Autodesk Inventor part; units mm, degrees
ref_plane "YZ Plane" through (0, 0, 0) normal (1, 0, 0) x (0, 1, 0)
ref_plane "XZ Plane" through (0, 0, 0) normal (0, 1, 0) x (-1, 0, 0)
ref_plane "XY Plane" through (0, 0, 0) normal (0, 0, 1) x (1, 0, 0)
ref_plane "Work Plane1" through (0, 0, 0) normal (0, 0, 1) x (1, 0, 0)
sketch "Sketch1" plane through (0, 0, 0) normal (0, 0, 1) x (1, 0, 0)
  line L0 (-150, -200) -> (150, -200)
  line L1 (150, -200) -> (150, 200)
  line L2 (150, 200) -> (-150, 200)
  line L3 (-150, 200) -> (-150, -200)
  line L4 (0, -280) -> (0, 280) construction
  line L5 (-210, 0) -> (210, 0) construction
  point P0 (0, 0)
  dimension "d0" = 400
  dimension "d1" = 300
extrude "Extrusion1" add sketch "Sketch1" against normal blind 12
sketch "Sketch2" plane through (0, 0, -12) normal (0, 0, 1) x (1, 0, 0)
  line L0 (0, 0) -> (-281.1142, 0) construction
  line L1 (0, 0) -> (0, -490.5016) construction
  line L2 (-150, -200) -> (150, -200) construction
  line L3 (-106.6853, -185) -> (102.3994, -185) construction
  line L4 (-96.6591, -157) -> (112.4256, -157) construction
  circle A0 centre (-82.5, -144) radius 2.15 construction
  circle A1 centre (-107.5, -144) radius 2.15 construction
  circle A2 centre (-107.5, 144) radius 2.15 construction
  circle A3 centre (-82.5, 144) radius 2.15 construction
  circle A4 centre (82.5, 144) radius 2.15 construction
  circle A5 centre (107.5, 144) radius 2.15 construction
  circle A6 centre (82.5, -144) radius 2.15 construction
  circle A7 centre (107.5, -144) radius 2.15 construction
  point P0 (-22.5, -157)
  point P1 (-34, -185)
  point P2 (22.5, -157)
  point P3 (34, -185)
  point P4 (-22.5, 157)
  point P5 (-34, 185)
  point P6 (34, 185)
  point P7 (22.5, 157)
  dimension "d8" = 15
  dimension "d9" = 28
  dimension "d10" = 22.5
  dimension "d11" = 34
hole "Hole2" at (-22.5, -157, -12) at (-34, -185, -12) at (34, -185, -12) at (22.5, -157, -12) at (-22.5, 157, -12) at (22.5, 157, -12) at (34, 185, -12) at (-34, 185, -12) at (107.5, -144, -12) at (82.5, -144, -12) at (-82.5, -144, -12) at (-107.5, -144, -12) at (-107.5, 144, -12) at (-82.5, 144, -12) at (82.5, 144, -12) at (107.5, 144, -12) direction (0, 0, 1) diameter 4.1 end through all counterbore diameter 7.2 counterbore depth 4.1
sketch "Sketch3" plane through (0, 0, -12) normal (0, 0, -1) x (-1, 0, 0)
  line L0 (-150, -200) -> (150, -200) construction
  line L1 (150, -200) -> (150, 200) construction
  line L2 (-150, 200) -> (-150, -200) construction
  line L3 (150, 200) -> (-150, 200) construction
  line L4 (135, -185) -> (-135, -185) construction
  line L5 (-135, -185) -> (-135, 185) construction
  line L6 (-135, 185) -> (135, 185) construction
  line L7 (135, 185) -> (135, -185) construction
  point P0 (0, 0)
  dimension "d29" = 15
hole "Hole3" at (-135, -185, -12) at (-135, 185, -12) at (135, 185, -12) at (135, -185, -12) direction (0, 0, 1) diameter 8.2 end through all
sketch "Sketch6" plane through (0, 0, -12) normal (0, 0, 1) x (1, 0, 0)
  line L0 (-27.5, -40) -> (27.5, -40) construction
  arc A0 (30.5, -43) -> (27.5, -40) centre (27.5, -43) ccw construction
  line L1 (30.5, -43) -> (30.5, -107) construction
  arc A1 (27.5, -110) -> (30.5, -107) centre (27.5, -107) ccw construction
  line L2 (27.5, -110) -> (-27.5, -110) construction
  arc A2 (-30.5, -107) -> (-27.5, -110) centre (-27.5, -107) ccw construction
  line L3 (-30.5, -107) -> (-30.5, -43) construction
  arc A3 (-27.5, -40) -> (-30.5, -43) centre (-27.5, -43) ccw construction
  circle A4 centre (-20.5, -75) radius 3.1 construction
  circle A5 centre (20.5, -50) radius 3.1 construction
  circle A6 centre (-20.5, -100) radius 3.1 construction
  circle A7 centre (-20.5, -50) radius 3.1 construction
  circle A8 centre (20.5, -100) radius 3.1 construction
  circle A9 centre (20.5, -75) radius 3.1 construction
hole "Hole6" at (-20.5, -100, -12) at (20.5, -100, -12) at (20.5, -75, -12) at (20.5, -50, -12) at (-20.5, -75, -12) at (-20.5, -50, -12) direction (0, 0, 1) diameter 6.2 end through all counterbore diameter 10.2 counterbore depth 6.2
properties part number "Metal_sheet" material "Aluminum 6061"
Geometry check sheet. Reference: the model listing, model coordinates, mm. A direction names the side the tool comes from. Coordinates: 2 decimals unless noted, no trailing zeros. One line per item, written item: value. Start each with the question number.
(1) Release check for a two-part mould opening along Y. For faces 1 (the face through (-2, -200, -6)), 2 (the face through (20.276, -105.095, -8.857)), 3 (the face through (2, 200, -6)) record: released by +Y, released by -Y, zero draft, split by the parting line, or undercut.
(2) Tool access check on faces 4 (the face through (-20.6, -71.7, -5.8)), 5 (the face through (132.229, 181.978, -5.916)). Record the directions out of +Z, -Z, +X, -X, +Y, -Y that give a thin tool (end or side, any length) a straight path to the whole face; none if there is none.
(3) Depth check by flat-ended pin: pin 1 (2 mm diameter, centred on x = -21, y = -155.5, fed in from -Z); pin 2 (3.5 mm diameter, centred on x = 107.5, y = -144, fed in from -Z); pin 3 (8 mm diameter, centred on x = 20.5, y = -100, fed in from -Z). Enter the tip coordinate at first touch or a pass-through.
(4) Scan lines: line 1 along X through (y, z) = (144, -10.1); line 2 along Y through (x, z) = (-33.5, -6.5); line 3 along X through (y, z) = (183.5, -6.75). Record each from-to range of solid material in increasing order. Write a range as [from, to].
Filled sheet:
1. face 1: released by -Y
1. face 2: undercut
1. face 3: released by +Y
2. face 4: -Z
2. face 5: +Z, -Z
3. pin 1: z = -7.9
3. pin 2: through
3. pin 3: z = -5.8
4. line 1: [-150, -111.1], [-103.9, -86.1], [-78.9, 78.9], [86.1, 103.9], [111.1, 150]
4. line 2: [-200, -186.99], [-183.01, 183.01], [186.99, 200]
4. line 3: [-150, -138.82], [-131.18, -35.4], [-32.6, 32.6], [35.4, 131.18], [138.82, 150]
